CAD build for the part. Positions are in the model's coordinates, mm. Give positions to 0.01 mm unless a question says otherwise; leave off trailing zeros. Order: outer loops, then holes, each group sorted by start corner. A loop starts at its lowest first (then second) coordinate and runs counter-clockwise, first axis right, second up.
Item 1: Band-saw the part on C-C on x = 40.5. Give the cut face in (y, z) (1 decimal).
Item 2: Wall check: L1, parallel to X at y = 48, z = 328; L2, parallel to Z at x = 18.5, y = 3 (3 decimals). Give the ranges that are in metal, low to high.
Item 3: Band-saw the part on A-A on z = 194.5. Give the cut face in (x, y), plus the area to 3 significant figures.
Item 4: Flat gauge pins, fed straight in: P1, Ø23, axis at x = 19, z = 158, coming from the +Y side; P2, Ø8, axis at y = 44, z = 310.5, coming from the +X side; P3, Ø4, axis at x = 6.5, y = 13.5, coming from the -Z side. Where does each tip first touch, or does it go through?
Item 5: Band-saw the part on B-B on y = 11. Give the cut face in (x, z) (1 decimal).
Autodesk Inventor part; units mm, degrees
ref_plane "YZ Plane" through (0, 0, 0) normal (1, 0, 0) x (0, 1, 0)
ref_plane "XZ Plane" through (0, 0, 0) normal (0, 1, 0) x (-1, 0, 0)
ref_plane "XY Plane" through (0, 0, 0) normal (0, 0, 1) x (1, 0, 0)
sketch "Sketch1" plane through (0, 0, 0) normal (0, 0, 1) x (1, 0, 0)
  line L0 (0, 0) -> (0, 50.8)
  line L1 (0, 50.8) -> (4.7625, 50.8)
  line L2 (4.7625, 50.8) -> (4.7625, 4.7625)
  line L3 (4.7625, 4.7625) -> (50.8, 4.7625)
  line L4 (50.8, 4.7625) -> (50.8, 0)
  line L5 (50.8, 0) -> (0, 0)
  dimension "d0" = 4.7625
  dimension "d1" = 50.8
  dimension "d2" = 4.7625
  dimension "d3" = 50.8
extrude "Extrusion1" add sketch "Sketch1" along normal blind 441.325
sketch "Sketch5" plane through (0, 0, 0) normal (0, -1, 0) x (1, 0, 0)
  line L0 (50.8, 441.325) -> (0, 441.325)
  line L1 (50.8, 0) -> (0, 0)
  line L2 (50.8, 0) -> (50.8, 441.325)
  line L3 (0, 441.325) -> (50.8, 390.525)
  line L4 (0, 0) -> (50.8, 50.8)
  dimension "d16" = 45
  dimension "d17" = 45
extrude "Extrusion5" cut sketch "Sketch5" against normal blind 50.8 contours L2 L3 L0
sketch "Sketch6" plane through (0, 0, 0) normal (0, -1, 0) x (1, 0, 0)
  line L0 (0, 0) -> (0, 441.325)
  line L1 (50.8, 0) -> (0, 0)
  line L2 (50.8, 0) -> (50.8, 390.525)
  line L3 (0, 0) -> (50.8, 50.8)
  dimension "d20" = 45
extrude "Extrusion6" cut sketch "Sketch6" against normal blind 50.8
properties part number "BOXC_L17P5"
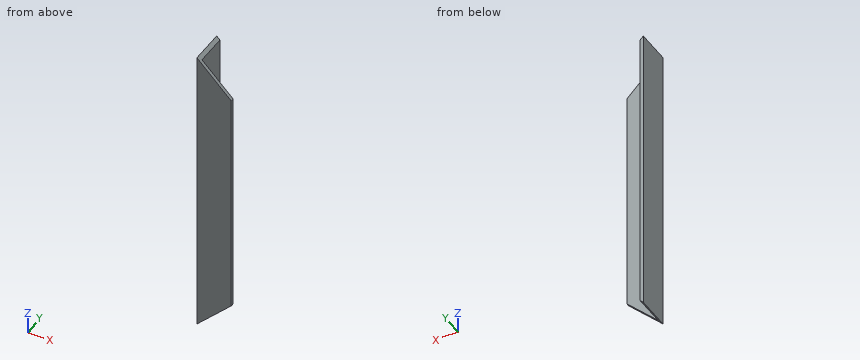
The answers:
1. outline: (0, 40.5) - (4.8, 40.5) - (4.8, 400.8) - (0, 400.8) - close
2. L1: x = 0 to 4.76
2. L2: z = 18.5 to 422.825
3. outline: (0, 0) - (50.8, 0) - (50.8, 4.76) - (4.76, 4.76) - (4.76, 50.8) - (0, 50.8) - close
3. area: 461 mm2
4. P1: stops at y = 4.76
4. P2: stops at x = 4.76
4. P3: stops at z = 4.5
5. outline: (0, 0) - (4.8, 4.8) - (4.8, 436.6) - (0, 441.3) - close
